Can you work these out from the model? Positions are in its coordinate system, mm. A direction names the side the tool comes from. Give positions to 0.01 mm unless a question says otherwise; leave off trailing zeros. Loops run counter-clockwise (first coordinate to the right, second up) from the corner with the lowest first, then second, coordinate; pieces in that order, holes last. Notation, with made-up numbers: (-13.75, -29) -> (4.25, -29) arc R3 cw to (4.25, -25) -> close; hole circle Ø10 at (-23, 52). An arc over 180 degrees is marked (long way). Return JSON: item names as keys, results as strings. Group by question number.
Q1. Will these pins go through, and if not, where does the flat tip stop? pin 1 (3 mm diameter, centred on y = 29, z = 3.5, fed in from +X); pin 2 (0.9 mm diameter, centred on x = -4.5, z = 5.5, fed in from -Y); pin 3 (2 mm diameter, centred on y = 3.5, z = -0.5, fed in from +X).
Q2. Thinking about a two-plate mould opening in Z: for faces 1 (the cylindrical face through (-4.4, 72.31, 0.11)), 2 (the cylindrical face through (-5.16, 2.89, 5.08)), 3 (the flat face through (-6, 36, -8)), which applies, pulls with the +Z half, pulls with the -Z half, needs draft (parallel to the pull), parting line crosses it, or undercut?
Q3. Which directions (+Z, -Z, +X, -X, +Y, -Y) give clear straight access to the entire face, cutting with the end or side of a thin tool? Please do faces 4 (the cylindrical face through (5.84, 2.58, -5.92)), 5 (the cylindrical face through (3.95, 75.26, -4.3)), 6 (the cylindrical face through (-1, 8.7, 0.1)), 7 (the flat face through (11, 75, 0)).
Q4. Suppose I cut it at D-D, the plane x = 0. Please give me the cut outline in (y, z), and give its area (3 significant figures).
Q5. I need wall thicknesses on line 1 along X through (y, z) = (3.2, -5.5); line 2 along Z through (x, y) = (6.5, 1.7); line 3 along Z through (x, y) = (4, 76.05). Which ranges of each line are inside material? Lowest first, please. Write a range as [from, to].
Q6. Suppose I cut it at A-A, the plane x = 6.5. Count the separate pieces of the cut face and the enclosed holes in it, and give its area (3 significant figures).
Autodesk Inventor part; units mm, degrees
ref_plane "Work Plane1" through (-12, 77.38, -8) normal (0, -1, 0) x (1, 0, 0)
ref_plane "YZ Plane" through (0, 0, 0) normal (1, 0, 0) x (0, 1, 0)
ref_plane "XZ Plane" through (0, 0, 0) normal (0, 1, 0) x (-1, 0, 0)
sketch "Sketch1" plane through (0, 0, 0) normal (0, 1, 0) x (-1, 0, 0)
  line L0 (9, 8) -> (-9, 8)
  line L1 (-9, 8) -> (-9, -8)
  line L2 (-9, -8) -> (9, -8)
  line L3 (9, -8) -> (9, 8)
  line L4 (9, 8) -> (-9, -8) construction
  line L5 (-9, 8) -> (9, -8) construction
  point P0 (0, 0)
  dimension "d0" = 18
  dimension "d1" = 16
extrude "Extrusion1" add sketch "Sketch1" along normal blind 4.5
ref_plane "Work Plane1" through (-12, 77.38, -8) normal (0, -1, 0) x (1, 0, 0)
sketch "Sketch6" plane through (0, 4.5, 0) normal (0, 1, 0) x (1, 0, 0)
  line L0 (9, 8) -> (-9, 8)
  line L1 (-9, -8) -> (9, -8)
  line L2 (-9, 8) -> (-5, 8)
  line L3 (-5, 8) -> (-5, -8)
  line L4 (-5, -8) -> (-9, -8)
  line L5 (-9, -8) -> (-9, 8)
  line L6 (9, -8) -> (9, 8)
  point P0 (0, 0)
  dimension "d27" = 14
extrude "WAZNE" add sketch "Sketch6" along normal up to surface (72.88 mm away) contours L3 L1 L5 L0
fillet "Fillet2" radius 14 1 edges at (-5, 4.5, 0)
sketch "Sketch7" plane through (0, 0, 0) normal (0, -1, 0) x (1, 0, 0)
  line L0 (-4.5, 5.5) -> (6.5, 5.5) construction
  line L1 (6.5, 5.5) -> (6.5, -5.5) construction
  line L2 (6.5, -5.5) -> (-4.5, -5.5) construction
  line L3 (-4.5, -5.5) -> (-4.5, 5.5) construction
  line L4 (9, 8) -> (9, -8)
  line L5 (-9, 8) -> (9, 8)
  point P0 (0, 0)
  dimension "d31" = 11
  dimension "d32" = 11
  dimension "d33" = 2.5
  dimension "d34" = 2.5
hole "Hole2" at (6.5, 0, 5.5) at (-4.5, 0, 5.5) at (-4.5, 0, -5.5) at (6.5, 0, -5.5) direction (0, 1, 0) diameter 1.567 depth 5.5
chamfer "Chamfer2" distance 0.2 angle 45 4 edges at (-4.5, 0, 6.2835) (6.5, 0, 6.2835) (6.5, 0, -4.7165) (-4.5, 0, -4.7165)
sketch "Sketch8" plane through (0, 77.38, 0) normal (0, 1, 0) x (1, 0, 0)
  line L0 (-9, 8) -> (-9, -8)
  line L1 (11, -8) -> (11, 8)
  line L2 (-9, 8) -> (11, 8)
  line L3 (11, 8) -> (11, -8)
  line L4 (11, -8) -> (-9, -8)
  line L5 (-9, -8) -> (-9, 8)
  point P0 (0, 0)
  point P1 (11, 8)
  dimension "d63" = 20
extrude "Extrusion6" add sketch "Sketch8" against normal blind 4.5
sketch "Sketch9" plane through (0, 72.88, 0) normal (0, -1, 0) x (1, 0, 0)
  line L0 (11, 8) -> (11, -8)
  line L1 (-5, -8) -> (-5, 8)
  line L2 (4, 7.0265) -> (4, -6.0756) construction
  point P0 (0, 0)
  point P1 (0, 0)
  point P2 (4, 5.5)
  point P3 (4, -5.5)
  dimension "d52" = 5
  dimension "d67" = 7
  dimension "d68" = 4
  dimension "d69" = 11
  dimension "d70" = 5.5
hole "Hole3" at (0, 72.88, 0) at (4, 72.88, 5.5) at (4, 72.88, -5.5) direction (0, 1, 0) diameter 2.4 end through all
chamfer "Chamfer3" distance 0.2 angle 45 3 edges at (0, 72.88, 1.2) (4, 72.88, 6.7) (4, 72.88, -4.3)
fillet "Fillet4" radius 2 1 edges at (-5, 72.88, 0)
properties part number "KN-00-02-09" material "X5CrNi18-10"
Ans:
{
 "1": {"pin 1": "stops at x = -5", "pin 2": "stops at y = 5.5", "pin 3": "stops at x = 9"},
 "2": {"face 1": "needs draft", "face 2": "undercut", "face 3": "pulls with the -Z half"},
 "3": {"face 4": "-Y", "face 5": "+Y", "face 6": "+Z, -Z, +X", "face 7": "+Z, -Z, +X, +Y, -Y"},
 "4": {"outline": "(0, -8) -> (7.78, -8) -> (7.78, 8) -> (0, 8) -> close; (72.88, -8) -> (77.38, -8) -> (77.38, -1.2) -> (73.08, -1.2) -> (72.88, -1.4) -> close; (72.88, 1.4) -> (73.08, 1.2) -> (77.38, 1.2) -> (77.38, 8) -> (72.88, 8) -> close", "area": "186 mm^2"},
 "5": {"line 1": "x = [-9, -5.28], [-3.72, 5.72], [7.28, 9]", "line 2": "z = [-8, -6.28], [-4.72, 4.72], [6.28, 8]", "line 3": "z = [-8, -6.7], [-4.3, 4.3], [6.7, 8]"},
 "6": {"separate pieces": "4", "enclosed holes": "0", "area": "133 mm^2"}
}
